Can you work these out from the model? Positions are in its coordinate system, mm. Coordinates: 2 decimals unless noted, no trailing zeros. Order: outer loops, then holes, each group sorted by start corner. A loop starts at its lowest first (then second) coordinate and runs counter-clockwise, first axis right, second up. Notation, with made-up numbers: (58.5, -7.75) -> (84.5, -7.75) arc R7 ccw to (84.5, -1.75) -> close; hole circle Ø6 at (64.25, -11.5). An arc over 180 degrees is marked (long way). Write item = value, one per line.
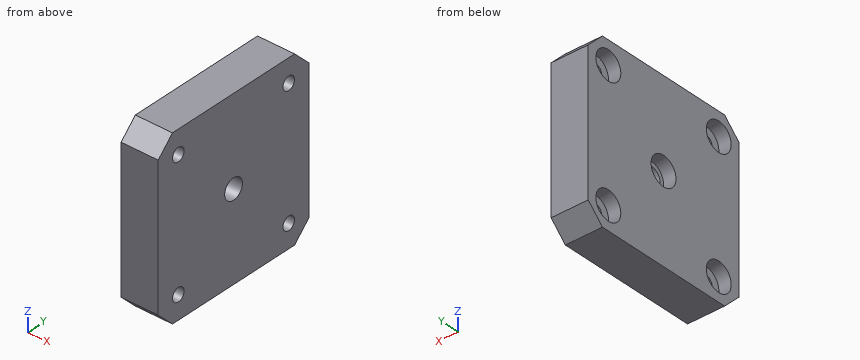
Autodesk Inventor part; units mm, degrees
ref_plane "YZ Plane" through (0, 0, 0) normal (1, 0, 0) x (0, 1, 0)
ref_plane "XZ Plane" through (0, 0, 0) normal (0, 1, 0) x (-1, 0, 0)
ref_plane "XY Plane" through (0, 0, 0) normal (0, 0, 1) x (1, 0, 0)
sketch "Skizze1" plane through (0, 0, 0) normal (1, 0, 0) x (0, 1, 0)
  line L0 (-29.61, 0) -> (29.61, 0)
  line L1 (0, -29.61) -> (0, 29.61)
  line L2 (-17.15, 21.15) -> (17.15, 21.15)
  line L3 (21.15, 17.15) -> (21.15, -17.15)
  line L4 (17.15, -21.15) -> (-17.15, -21.15)
  line L5 (-21.15, -17.15) -> (-21.15, 17.15)
  line L6 (21.15, 17.15) -> (17.15, 21.15)
  line L7 (21.15, -17.15) -> (17.15, -21.15)
  line L8 (-17.15, -21.15) -> (-21.15, -17.15)
  line L9 (-17.15, 21.15) -> (-21.15, 17.15)
  circle A0 centre (0, 0) radius 2.5
  point P0 (-21.15, 21.15)
  point P1 (21.15, -21.15)
  point P2 (21.15, 21.15)
  point P3 (-21.15, -21.15)
  dimension "d0" = 42.3
  dimension "d1" = 42.3
  dimension "d5" = 4
  dimension "d6" = 4
  dimension "d7" = 4
  dimension "d8" = 4
  dimension "d9" = 4
  dimension "d10" = 4
  dimension "d11" = 4
  dimension "d12" = 4
  dimension "d13" = 5
extrude "Extrusion2" add sketch "Skizze1" along normal mid plane 9 contours L5 L9 L2 L1 A0 L0 | L0 A0 L1 L4 L8 L5 | L1 L2 L6 L3 L0 A0 | A0 L0 L3 L7 L4 L1
sketch "Skizze2" plane through (4.5, 0, 0) normal (1, 0, 0) x (0, 0, -1)
  circle A0 centre (0, 0) radius 2.5
  line L0 (-17.15, 21.15) -> (-21.15, 17.15)
  line L1 (-21.15, 17.15) -> (-21.15, -17.15)
  line L2 (-21.15, -17.15) -> (-17.15, -21.15)
  line L3 (-17.15, -21.15) -> (17.15, -21.15)
  line L4 (17.15, -21.15) -> (21.15, -17.15)
  line L5 (21.15, -17.15) -> (21.15, 17.15)
  line L6 (21.15, 17.15) -> (17.15, 21.15)
  line L7 (17.15, 21.15) -> (-17.15, 21.15)
  line L8 (0, -29.61) -> (0, 29.61)
  line L9 (29.61, 0) -> (-29.61, 0)
  point P0 (-15.5, 15.5)
  point P1 (15.5, 15.5)
  point P2 (-15.5, -15.5)
  point P3 (15.5, -15.5)
  dimension "d18" = 15.5
  dimension "d19" = 15.5
hole "Bohrung1" at (4.5, 15.5, 15.5) at (4.5, 15.5, -15.5) at (4.5, -15.5, 15.5) at (4.5, -15.5, -15.5) direction (-1, 0, 0) diameter 3.242 end through all
sketch "Skizze4" plane through (-4.5, 0, 0) normal (-1, 0, 0) x (0, 0, 1)
  circle A0 centre (15.5, -15.5) radius 1.621
  circle A1 centre (15.5, 15.5) radius 1.621
  circle A2 centre (-15.5, 15.5) radius 1.621
  circle A3 centre (-15.5, -15.5) radius 1.621
  circle A4 centre (0, 0) radius 2.5
  line L0 (21.15, 17.15) -> (17.15, 21.15)
  line L1 (17.15, 21.15) -> (-17.15, 21.15)
  line L2 (-17.15, 21.15) -> (-21.15, 17.15)
  line L3 (-21.15, 17.15) -> (-21.15, -17.15)
  line L4 (-21.15, -17.15) -> (-17.15, -21.15)
  line L5 (-17.15, -21.15) -> (17.15, -21.15)
  line L6 (17.15, -21.15) -> (21.15, -17.15)
  line L7 (21.15, -17.15) -> (21.15, 17.15)
  circle A5 centre (15.5, 15.5) radius 3.5
  circle A6 centre (15.5, -15.5) radius 3.5
  circle A7 centre (-15.5, 15.5) radius 3.5
  circle A8 centre (-15.5, -15.5) radius 3.5
  dimension "d34" = 7
  dimension "d35" = 7
  dimension "d36" = 7
  dimension "d37" = 7
extrude "Extrusion4" cut sketch "Skizze4" against normal blind 3 contours A5 | A6 | A7 | A8
sketch "Skizze5" plane through (-4.5, 0, 0) normal (-1, 0, 0) x (0, 0, 1)
  circle A0 centre (-15.5, 15.5) radius 3.5
  circle A1 centre (15.5, 15.5) radius 3.5
  circle A2 centre (15.5, -15.5) radius 3.5
  circle A3 centre (-15.5, -15.5) radius 3.5
  circle A4 centre (0, 0) radius 2.5
  line L0 (21.15, 17.15) -> (17.15, 21.15)
  line L1 (17.15, 21.15) -> (-17.15, 21.15)
  line L2 (-17.15, 21.15) -> (-21.15, 17.15)
  line L3 (-21.15, 17.15) -> (-21.15, -17.15)
  line L4 (-21.15, -17.15) -> (-17.15, -21.15)
  line L5 (-17.15, -21.15) -> (17.15, -21.15)
  line L6 (17.15, -21.15) -> (21.15, -17.15)
  line L7 (21.15, -17.15) -> (21.15, 17.15)
  circle A5 centre (0, 0) radius 3.5
  dimension "d40" = 7
extrude "Extrusion5" cut sketch "Skizze5" against normal blind 3 contours A5
properties part number "BackPlatte" material "Stahl, Kohlenstoff"
Item 1: If I drill on probe 1 along Y at (x, z) = (-3.3, 15.5); probe 2 along Y at (x, z) = (3.15, 15.5); probe 3 along Y at (x, z) = (-2.4, 0), over which ranges is the centre line in solid material (lowest first)?
A:
probe_1 = -21.15 to -19, -12 to 12, 19 to 21.15
probe_2 = -21.15 to -17.12, -13.88 to 13.88, 17.12 to 21.15
probe_3 = -21.15 to -3.5, 3.5 to 21.15
Item 2: I want a section at A-A, the plane y = 0. Please give me the cut outline in (x, z), plus the area to 3 significant figures.
A:
outline = (-4.5, -21.15) -> (4.5, -21.15) -> (4.5, -2.5) -> (-1.5, -2.5) -> (-1.5, -3.5) -> (-4.5, -3.5) -> close; (-4.5, 3.5) -> (-1.5, 3.5) -> (-1.5, 2.5) -> (4.5, 2.5) -> (4.5, 21.15) -> (-4.5, 21.15) -> close
area = 330 mm2
Item 3: I want a section at B-B, the plane z = -15.5. Please give me the cut outline in (x, y), plus the area to 3 significant figures.
A:
outline = (-4.5, -21.15) -> (4.5, -21.15) -> (4.5, -17.12) -> (-1.5, -17.12) -> (-1.5, -19) -> (-4.5, -19) -> close; (-4.5, -12) -> (-1.5, -12) -> (-1.5, -13.88) -> (4.5, -13.88) -> (4.5, 13.88) -> (-1.5, 13.88) -> (-1.5, 12) -> (-4.5, 12) -> close; (-4.5, 19) -> (-1.5, 19) -> (-1.5, 17.12) -> (4.5, 17.12) -> (4.5, 21.15) -> (-4.5, 21.15) -> close
area = 300 mm2
Item 4: I'm going to push a flat-ended pin straight in: P1, Ø5, axis at y = -15.5, z = -15.5, coming from the -X side. Where does the tip first touch, or does it pass through?
A:
P1 = -1.5
Item 5: I want a section at C-C, the plane x = -1. Please give me the cut outline in (y, z), plus the area to 3 significant figures.
A:
outline = (-21.15, -17.15) -> (-17.15, -21.15) -> (17.15, -21.15) -> (21.15, -17.15) -> (21.15, 17.15) -> (17.15, 21.15) -> (-17.15, 21.15) -> (-21.15, 17.15) -> close; hole circle Ø3.24 at (-15.5, -15.5); hole circle Ø3.24 at (-15.5, 15.5); hole circle Ø5 at (0, 0); hole circle Ø3.24 at (15.5, -15.5); hole circle Ø3.24 at (15.5, 15.5)
area = 1,700 mm2
